from build123d import *

# Parameters (mm, degrees)
SKETCH_1_W          = 68
SKETCH_1_H          = 58
SKETCH_1_R          = 1.25
EXTRUDE_1_DEPTH     = 2
SKETCH_2_W          = 2
SKETCH_2_H          = 40
EXTRUDE_2_DEPTH     = 68
SKETCH_3_W          = 14
SKETCH_3_H          = 25
CUT_EXTRUDE_1_DEPTH = 10
FILLET_1_R          = 2


with BuildPart() as part:
    # 草图1 → 凸台-拉伸1 (new body)
    with BuildSketch(Plane.XY):
        with Locations((34, 29)):
            Rectangle(SKETCH_1_W, SKETCH_1_H)
        with Locations((48, 27)):
            Circle(SKETCH_1_R, mode=Mode.SUBTRACT)
        with Locations(Location((20, 27, 0), (0, 0, 180))):
            Circle(SKETCH_1_R, mode=Mode.SUBTRACT)
        with Locations((48, 47)):
            Circle(SKETCH_1_R, mode=Mode.SUBTRACT)
        with Locations(Location((20, 47, 0), (0, 0, 180))):
            Circle(SKETCH_1_R, mode=Mode.SUBTRACT)
    extrude(amount=EXTRUDE_1_DEPTH)

    # 草图2 → 凸台-拉伸2 (add)
    with BuildSketch(Plane(origin=(68, 0, 0), x_dir=(0, 0, -1), z_dir=(1, 0, 0))):
        with Locations((-1, -20)):
            Rectangle(SKETCH_2_W, SKETCH_2_H)
    extrude(amount=-EXTRUDE_2_DEPTH)

    # 草图3 → 切除-拉伸1 (cut)
    with BuildSketch(Plane.XY.offset(2)):
        with Locations((61, -27.5)):
            Rectangle(SKETCH_3_W, SKETCH_3_H)
        with Locations((7, -27.5)):
            Rectangle(SKETCH_3_W, SKETCH_3_H)
    extrude(amount=-CUT_EXTRUDE_1_DEPTH, mode=Mode.SUBTRACT)

    # 圆角1
    fillet_1_edges = [part.edges().sort_by_distance(p)[0] for p in [
        (54, -15, 1),
        (14, -15, 1),
    ]]
    fillet(fillet_1_edges, radius=FILLET_1_R)


solid = part.part
Part model, mm, in its own coordinate system. A direction names the side the tool comes from. Give positions to 0.01 mm unless a question says otherwise; leave off trailing zeros. Order: outer loops, then holes, each group sorted by start corner. A loop starts at its lowest first (then second) coordinate and runs counter-clockwise, first axis right, second up. Notation, with made-up numbers: (-6.75, 7.5) - (21.25, 7.5) arc R25 ccw to (21.25, 31.5) - close; hole circle Ø11 at (18, 12). An arc over 180 degrees is marked (long way). Use a Markdown table: item, result.
1) Saw through at D-D on x = 11. List the corners of the cut face in (y, z).
Checked values:
| item | result |
|---|---|
| outline | (-15, 0) - (58, 0) - (58, 2) - (-15, 2) - close |
2) Two-plate mould, pull along Y, no slides. Class faces 1 (the cylindrical face through (47.84, 48.24, 0.99)), 2 (the cylindrical face through (13.4, -15.57, 0.99)), 3 (the flat face through (0, 22, 1)): +Y half, -Y half, draft (parallel to the pull), parting line (faces both ways), or undercut.
Checked values:
| item | result |
|---|---|
| face 1 | undercut |
| face 2 | -Y half |
| face 3 | draft |
3) Saw through at A-A on x = 48. List the corners of the cut face in (y, z).
Checked values:
| item | result |
|---|---|
| outline | (-40, 0) - (25.75, 0) - (25.75, 2) - (-40, 2) - close; (28.25, 0) - (45.75, 0) - (45.75, 2) - (28.25, 2) - close; (48.25, 0) - (58, 0) - (58, 2) - (48.25, 2) - close |
4) 3-axis set-ups, long thin cutter, end or side, ignore diameter. For faces 4 (the cylindrical face through (18.845, 27.479, 0.986)), 5 (the flat face through (62, -15, 1)), 6 (the flat face through (6, -15, 1)): which of +Z, -Z, +X, -X, +Y, -Y reach the whole face in a straight line?
Checked values:
| item | result |
|---|---|
| face 4 | +Z, -Z |
| face 5 | +Z, -Z, +X, -Y |
| face 6 | +Z, -Z, -X, -Y |
5) Saw through at B-B on y = 27. List the corners of the cut face in (x, z).
Checked values:
| item | result |
|---|---|
| outline | (0, 0) - (18.75, 0) - (18.75, 2) - (0, 2) - close; (21.25, 0) - (46.75, 0) - (46.75, 2) - (21.25, 2) - close; (49.25, 0) - (68, 0) - (68, 2) - (49.25, 2) - close |
6) Flat gauge pins, fed straight in: P1, Ø1, axis at y = -26.5, z = 1, coming from the +X side; P2, Ø1, axis at y = -32.5, z = 1.5, coming from the -X side. Where does each tip first touch, or does it go through?
Checked values:
| item | result |
|---|---|
| P1 | x = 54 |
| P2 | x = 14 |
7) Saw through at C-C on z = 1.55. List the corners of the cut face in (x, y).
Checked values:
| item | result |
|---|---|
| outline | (0, -15) - (12, -15) arc R2 cw to (14, -17) - (14, -40) - (54, -40) - (54, -17) arc R2 cw to (56, -15) - (68, -15) - (68, 58) - (0, 58) - close; hole circle Ø2.5 at (20, 27); hole circle Ø2.5 at (20, 47); hole circle Ø2.5 at (48, 27); hole circle Ø2.5 at (48, 47) |
8) Probe L1, parallel to Y at x = 20, z = 0.95; L2, parallel to X at y = 28, z = 1.05; L3, parallel to X at y = -24, z = 1.65. List the from-to ranges inside material, lowest first. Write a range as from..to.
Checked values:
| item | result |
|---|---|
| L1 | -40..25.75, 28.25..45.75, 48.25..58 |
| L2 | 0..19.25, 20.75..47.25, 48.75..68 |
| L3 | 14..54 |
